```python
from build123d import *

# Parameters (mm, degrees)
SKETCH_1_W                  = 8
SKETCH_1_H                  = 50
EXTRUDE_1_DEPTH             = 97
HOLE_WIZARD_M5_2_AT_2_COUNT = 2
HOLE_WIZARD_M5_2_AT_2_PITCH = 30
HOLE_WIZARD_M3_1_D          = 2.5
HOLE_WIZARD_M3_1_DEPTH      = 7.5
HOLE_WIZARD_M3_1_TIP        = 0.751075774


with BuildPart() as part:
    # 草图1 → 凸台-拉伸1 (new body)
    with BuildSketch(Plane.XY):
        with Locations((4, 25)):
            Rectangle(SKETCH_1_W, SKETCH_1_H)
    extrude(amount=EXTRUDE_1_DEPTH)

    # 草图6 → M5 螺纹孔2 (revolve, cut)
    with BuildSketch(Plane(origin=(4, 40, 0), x_dir=(0, 1, 0), z_dir=(1, 0, 0))):
        Polygon((0, 0), (0, 13.6618073), (2.1, 12.4), (2.1, 0), align=None)
    hole_wizard_m5_2 = revolve(axis=Axis((4, 40, -6.35), (0, 0, 1)), mode=Mode.SUBTRACT)

    # M5 螺纹孔2 at 2: M5 螺纹孔2 ×2
    with Locations(*[(0, -i * HOLE_WIZARD_M5_2_AT_2_PITCH, 0) for i in range(1, HOLE_WIZARD_M5_2_AT_2_COUNT)]):
        add(hole_wizard_m5_2, mode=Mode.SUBTRACT)

    # 镜向1: M5 螺纹孔2 across plane
    add(hole_wizard_m5_2.mirror(Plane(origin=(0, 0, 48.5), x_dir=(1, 0, 0), z_dir=(0, 0, -1))), mode=Mode.SUBTRACT)

    # 镜向1 copy 1 sketch → 镜向1 copy 1 (revolve, cut)
    with BuildSketch(Plane(origin=(4, 10, 97), x_dir=(0, 1, 0), z_dir=(1, 0, 0))):
        Polygon((0, 0), (0, -13.6618073), (2.1, -12.4), (2.1, 0), align=None)
    revolve(axis=Axis((4, 10, 103.35), (0, 0, 1)), mode=Mode.SUBTRACT)

    # M3 螺纹孔1
    with Locations(Plane(origin=(0, 50, 0), x_dir=(1, 0, 0), z_dir=(0, 1, 0))):
        with Locations((4, -71.5), (4, -52.5)):
            Hole(HOLE_WIZARD_M3_1_D / 2, depth=HOLE_WIZARD_M3_1_DEPTH)
            with Locations((0, 0, -(HOLE_WIZARD_M3_1_DEPTH + HOLE_WIZARD_M3_1_TIP / 2))):  # 118° drill point
                Cone(0, HOLE_WIZARD_M3_1_D / 2, HOLE_WIZARD_M3_1_TIP, mode=Mode.SUBTRACT)


solid = part.part
```
Design review of the part built by this model. Coordinates are the model's own, in mm. A direction names the side the tool comes from. Round coordinates to 2 decimals unless told otherwise and drop trailing zeros. Order: outer loops, then holes, each group sorted by start corner. A loop starts at its lowest first (then second) coordinate and runs counter-clockwise, first axis right, second up. Notation, with made-up numbers: (82.5, 80) - (128.5, 80) arc R11 ccw to (128.5, 95) - close; hole circle Ø1 at (21, 82.5). An arc over 180 degrees is marked (long way). One line per question, with ' | ' between items.
Item 1: Draft analysis for pull direction Y (two halves, no side actions). For faces 1 (the face through (3.75, 39.73, 83.56)), 2 (the face through (4, 25, 0)), 3 (the face through (3.972, 41.879, 71.285)), state which applies: +Y half, -Y half, draft (parallel to the pull), parting line (faces both ways), or undercut.
Checks:
face 1: undercut | face 2: draft | face 3: +Y half
Item 2: Wall thickness on line 1 (Z direction, x = 4, y = 45.75); line 2 (Y direction, x = 4, z = 87.5); line 3 (X direction, y = 40, z = 88): over which ranges is each line inside the solid? List them lowest first. Write a range as [from, to].
Checks:
line 1: [0, 51.25], [53.75, 70.25], [72.75, 97] | line 2: [0, 7.9], [12.1, 37.9], [42.1, 50] | line 3: [0, 1.9], [6.1, 8]
Item 3: Take a section at A-A, the plane z = 8. Write out the cut boundary in (x, y).
Checks:
outline: (0, 0) - (8, 0) - (8, 50) - (0, 50) - close; hole circle Ø4.2 at (4, 10); hole circle Ø4.2 at (4, 40)
Item 4: For P1, Ø2.5, axis at x = 4, y = 10, coming from the -Z side, flat-tipped, find the tip position at first contact; note if it passes through.
Checks:
P1: z = 12.91
Item 5: Machinability: for faces 4 (the face through (5.278, 8.334, 90.887)), 5 (the face through (4.16, 46.2, 70.26)), 6 (the face through (5.278, 8.334, 6.113)), which of the approach directions +Z, -Z, +X, -X, +Y, -Y give a long, thin tool a straight path to every point of the face, cutting with its end or side? Answer none if there is none.
Checks:
face 4: +Z | face 5: +Y | face 6: -Z
